Can you work these out from the model? Positions are in its coordinate system, mm. A direction names the side the tool comes from. Coordinates: 2 decimals unless noted, no trailing zeros.
```python
from build123d import *

# Parameters (mm, degrees)
SKETCH1_W           = 256.794
SKETCH1_H           = 196.85
BOSS_EXTRUDE1_DEPTH = 12.7
SKETCH2_W           = 10.16
SKETCH2_H           = 25.4
CUT_EXTRUDE1_DEPTH  = 12.7
SKETCH3_R           = 3.81
CUT_EXTRUDE2_DEPTH  = 12.7
SKETCH4_W           = 256.794
SKETCH4_H           = 12.7
BOSS_EXTRUDE2_DEPTH = 12.7


with BuildPart() as part:
    # Sketch1 → Boss-Extrude1 (new body)
    with BuildSketch(Plane.XY):
        with Locations((50.169769953, -9.226877934)):
            Rectangle(SKETCH1_W, SKETCH1_H)
    extrude(amount=BOSS_EXTRUDE1_DEPTH)

    # Sketch2 → Cut-Extrude1 (cut)
    with BuildSketch(Plane(origin=(178.566769953, 0, 0), x_dir=(0, 0, -1), z_dir=(1, 0, 0))):
        with Locations((-6.35, -12.393940124)):
            Rectangle(SKETCH2_W, SKETCH2_H)
    extrude(amount=-CUT_EXTRUDE1_DEPTH, mode=Mode.SUBTRACT)

    # Sketch3 → Cut-Extrude2 (cut)
    with BuildSketch(Plane.XY.offset(12.7)):
        with Locations((172.216769953, -6.043940124)):
            Circle(SKETCH3_R)
        with Locations((172.216769953, -18.743940124)):
            Circle(SKETCH3_R)
    extrude(amount=-CUT_EXTRUDE2_DEPTH, mode=Mode.SUBTRACT)

    # Sketch4 → Boss-Extrude2 (add)
    with BuildSketch(Plane(origin=(0, 89.198122066, 0), x_dir=(1, 0, 0), z_dir=(0, 1, 0))):
        with Locations((50.169769953, -6.35)):
            Rectangle(SKETCH4_W, SKETCH4_H)
    extrude(amount=BOSS_EXTRUDE2_DEPTH)


solid = part.part
```
1. I'm going to push a flat-ended pin straight in: pin 1 (4 mm diameter, centred on x = 170.5, y = -6.5, fed in from +Z). Where does the tip first touch, or does it pass through?
Completed:
pin 1: passes through
2. Please list where this line runs through material, in increasing order: probe 1 along X at (y, z) = (-2, 10.25).
Completed:
probe 1: x = -78.23 to 165.87
3. On a 3-axis mill with a long thin cutter (end or side, diameter ignored), from which of +Z, -Z, +X, -X, +Y, -Y can I reach the whole of each face in a straight line? I mean faces 5 (the cylindrical face through (175.736, -7.503, 12.074)), 6 (the flat face through (165.867, -12, 6)). Say none if no direction works.
Completed:
face 5: +Z, -Z
face 6: +X
4. Thinking about a two-plate mould opening in Z: for faces 1 (the flat face through (48, -4, 0)), 2 (the flat face through (172, -25.094, 6)), 3 (the flat face through (172, -13, 11.43)), 4 (the cylindrical face through (175.736, -7.503, 0.644)), which applies, pulls with the +Z half, pulls with the -Z half, needs draft (parallel to the pull), parting line crosses it, or undercut?
Completed:
face 1: pulls with the -Z half
face 2: undercut
face 3: undercut
face 4: needs draft
